from build123d import *

# Parameters (mm, degrees)
F1_DEPTH  = 74.8970308
F2_R      = 1.35255
F3_DEPTH  = 1.70942
F8_DEPTH  = 150.2936248359
F10_DEPTH = 91.0812758
F11_R     = 3.69315
F12_R     = 1.98373
F12_R_2   = 1.98374
F13_R     = 0.762


# Not quite as in the source:
# - a fillet or chamfer is up to 0.001 mm smaller than in the source, because OpenCascade refuses the exact size


with BuildPart() as f1:
    # F0 (on Top) → F1 (new body)
    with BuildSketch(Plane.XY):
        Polygon((0, -34.9127429517), (0, 0), (4.6326774961, 3.932751029), (7.9712502047, 0), (9.2744217668, 1.1062823402), (4.8295667179, 6.3422049313), (-1.70942, 0.7911587457), (-1.70942, -36.6221629517), (155.9705248359, -36.6221629517), (155.9705248359, 0.7911587457), (149.4315381179, 6.3422049313), (144.9866830691, 1.1062823402), (146.2898546311, 0), (149.6284273398, 3.932751029), (154.2611048359, 0), (154.2611048359, -34.9127429517), align=None)
    extrude(amount=F1_DEPTH)

    # F2 (on face) → F3 (cut, through all)
    with BuildSketch(Plane(origin=(0, -34.9127429517, 0), x_dir=(-1, 0, 0), z_dir=(0, 1, 0))):
        with Locations((-5.15874, 3.175)):
            Circle(F2_R)
        with Locations((-5.15874, 63.2981208)):
            Circle(F2_R)
        with Locations((-149.1023648359, 63.2981208)):
            Circle(F2_R)
        with Locations((-149.1023648359, 3.175)):
            Circle(F2_R)
    extrude(amount=-F3_DEPTH, mode=Mode.SUBTRACT)

    # F7 (on offset) → F8 (join, through all)
    with BuildSketch(Plane.YZ.offset(1.98374)):
        with BuildLine():
            Line((-36.6221629517, 74.8970308), (-34.9127429517, 74.8970308))
            ThreePointArc((-34.9127429517, 74.8970308), (-35.0846656967, 76.2029136969), (-35.5887176805, 77.4198028324))
            Line((-35.5887176805, 77.4198028324), (-81.129350806, 156.2984932146))
            Line((-81.129350806, 156.2984932146), (-82.6097519517, 155.4437832146))
            Line((-82.6097519517, 155.4437832146), (-37.0691188262, 76.5650928324))
            ThreePointArc((-37.0691188262, 76.5650928324), (-36.7358386226, 75.7604832448), (-36.6221629517, 74.8970308))
        make_face()
    extrude(amount=F8_DEPTH)

    # F9 (on face) → F10 (join)
    with BuildSketch(Plane(origin=(0, -87.96157055, 152.3539093062), x_dir=(1, 0, 0), z_dir=(0, -0.5, 0.8660254038))):
        Polygon((-1.7094199999, 6.1797478168), (1.98374, 6.1797478168), (1.98374, 7.8891678168), (0, 7.8891678168), (1e-10, 28.9964815425), (4.3557372213, 33.3522187635), (8.0035172575, 29.7044387269), (9.2122597315, 30.9131812007), (4.3557372215, 35.7697037112), (-1.7094199999, 29.7045464903), align=None)
        Polygon((152.277364836, 7.8891678168), (152.277364836, 6.1797478168), (155.9705248359, 6.1797478168), (155.9705248359, 29.7045464903), (149.9053676148, 35.7697037114), (145.0488451045, 30.9131812012), (146.2575875784, 29.7044387273), (149.9053676148, 33.3522187636), (154.2611048359, 28.9964815425), (154.2611048359, 7.8891678168), align=None)
    extrude(amount=-F10_DEPTH)

    # F11 (radius 3.69316 in the source; OpenCascade refuses exactly that, so slightly less here)
    f11_edges = [f1.edges().sort_by_distance(p)[0] for p in [
        (149.431538, 6.342205, 37.448515),
        (155.970525, 0.791159, 37.448515),
        (155.970525, -36.622163, 37.448515),
        (-1.70942, -36.622163, 37.448515),
        (-1.70942, 0.791159, 37.448515),
        (4.829567, 6.342205, 37.448515),
        (149.905368, -34.21378, 130.799412),
        (155.970525, -39.46636, 127.766833),
        (155.970525, -59.839433, 116.004434),
        (-1.70942, -59.839433, 116.004434),
        (-1.70942, -39.46636, 127.766833),
        (4.355737, -34.21378, 130.799412),
    ]]
    fillet(f11_edges, radius=F11_R)

    # F12#9 (call 1 of 12: OpenCascade refuses the feature's edges together) (radius 1.98374 in the source; OpenCascade refuses exactly that, so slightly less here)
    f12_9_edges = [f1.edges().sort_by_distance(p)[0] for p in [
        (0, -58.359032, 116.859144),
    ]]
    fillet(f12_9_edges, radius=F12_R)

    # F12#10 (call 2 of 12) (radius 1.98374 in the source; OpenCascade refuses exactly that, so slightly less here)
    f12_10_edges = [f1.edges().sort_by_distance(p)[0] for p in [
        (154.261105, -58.359032, 116.859144),
    ]]
    fillet(f12_10_edges, radius=F12_R)

    # F12#11 (call 3 of 12)
    f12_11_edges = [f1.edges().sort_by_distance(p)[0] for p in [
        (154.261105, -40.079562, 127.412801),
    ]]
    fillet(f12_11_edges, radius=F12_R_2)

    # F12#12 (call 4 of 12)
    f12_12_edges = [f1.edges().sort_by_distance(p)[0] for p in [
        (149.905368, -36.307383, 129.590669),
    ]]
    fillet(f12_12_edges, radius=F12_R_2)

    # F12 (call 5 of 12)
    f12_edges = [f1.edges().sort_by_distance(p)[0] for p in [
        (149.628427, 3.932751, 37.448515),
    ]]
    fillet(f12_edges, radius=F12_R_2)

    # F12#2 (call 6 of 12)
    f12_2_edges = [f1.edges().sort_by_distance(p)[0] for p in [
        (154.261105, 0, 37.448515),
    ]]
    fillet(f12_2_edges, radius=F12_R_2)

    # F12#3 (call 7 of 12)
    f12_3_edges = [f1.edges().sort_by_distance(p)[0] for p in [
        (154.261105, -34.912743, 37.448515),
    ]]
    fillet(f12_3_edges, radius=F12_R_2)

    # F12#4 (call 8 of 12)
    f12_4_edges = [f1.edges().sort_by_distance(p)[0] for p in [
        (0, -34.912743, 37.448515),
    ]]
    fillet(f12_4_edges, radius=F12_R_2)

    # F12#5 (call 9 of 12)
    f12_5_edges = [f1.edges().sort_by_distance(p)[0] for p in [
        (0, 0, 37.448515),
    ]]
    fillet(f12_5_edges, radius=F12_R_2)

    # F12#6 (call 10 of 12)
    f12_6_edges = [f1.edges().sort_by_distance(p)[0] for p in [
        (4.632677, 3.932751, 37.448515),
    ]]
    fillet(f12_6_edges, radius=F12_R_2)

    # F12#7 (call 11 of 12)
    f12_7_edges = [f1.edges().sort_by_distance(p)[0] for p in [
        (0, -40.079562, 127.412801),
    ]]
    fillet(f12_7_edges, radius=F12_R_2)

    # F12#8 (call 12 of 12)
    f12_8_edges = [f1.edges().sort_by_distance(p)[0] for p in [
        (4.355737, -36.307383, 129.590669),
    ]]
    fillet(f12_8_edges, radius=F12_R_2)

    # F13
    f13_edges = [f1.edges().sort_by_distance(p)[0] for p in [
        (145.638269, 0.553141, 74.897031),
        (145.638269, 0.553141, 0),
        (8.622836, 0.553141, 0),
        (8.622836, 0.553141, 74.897031),
        (8.607888, -61.713371, 167.508314),
        (8.607888, -16.172733, 88.629616),
        (145.653216, -16.172733, 88.629616),
        (145.653216, -61.713371, 167.508314),
    ]]
    fillet(f13_edges, radius=F13_R)


solid = f1.part
Can you work these out from the model? Positions are in its coordinate system, mm. A direction names the side the tool comes from. Round coordinates to 2 decimals unless told otherwise and drop trailing zeros. Order: outer loops, then holes, each group sorted by start corner. A loop starts at its lowest first (then second) coordinate and runs counter-clockwise, first axis right, second up. Notation, with made-up numbers: M 61.5,33 L 76.5,33 A24 ccw 76.5,56 Z; hole C -7.75,54 d8. An arc over 180 degrees is marked long. Use a Markdown table: item, result.
1) Imagine slicing it at C-C (x = 110). List the corners of the cut face in (y, z) for me, then the cut area to 3 significant figures.
Geometry says:
| item | result |
|---|---|
| outline | M -82.61,155.44 L -37.07,76.57 A3.34 cw -36.62,74.9 L -36.62,0 L -34.91,0 L -34.91,74.9 A5.05 ccw -35.59,77.42 L -81.13,156.3 Z |
| area | 287 mm² |
2) If we mould it in two halves opening along Z, with no side actions, what happens to faces 4 (the face through (-0.6, -58.61, 115.98)), 5 (the face through (154.261, -49, 123)), 6 (the face through (0, -49, 123)), 7 (the face through (154.261, -17, 37))? For each: +Z half, -Z half, draft (parallel to the pull), parting line (faces both ways), or undercut.
Geometry says:
| item | result |
|---|---|
| face 4 | -Z half |
| face 5 | undercut |
| face 6 | undercut |
| face 7 | draft |
3) Imagine slicing it at A-A (z = 35). List the corners of the cut face in (x, y) for me, then the cut area to 3 significant figures.
Geometry says:
| item | result |
|---|---|
| outline | M -1.71,-32.93 A3.69 ccw 1.98,-36.62 L 152.28,-36.62 A3.69 ccw 155.97,-32.93 L 155.97,-0.92 A3.69 ccw 154.67,1.9 L 152.25,3.95 A3.69 ccw 147.04,3.53 L 144.99,1.11 L 146.29,0 L 148.34,2.42 A1.98 cw 151.14,2.65 L 153.56,0.59 A1.98 cw 154.26,-0.92 L 154.26,-32.93 A1.98 cw 152.28,-34.91 L 1.98,-34.91 A1.98 cw 0,-32.93 L 0,-0.92 A1.98 cw 0.7,0.59 L 3.12,2.65 A1.98 cw 5.92,2.42 L 7.97,0 L 9.27,1.11 L 7.22,3.53 A3.69 ccw 2.01,3.95 L -0.41,1.9 A3.69 ccw -1.71,-0.92 Z |
| area | 427 mm² |
4) On a 3-axis mill with a long thin cutter (end or side, diameter ignored), from which of +Z, -Z, +X, -X, +Y, -Y can I reach the whole of each face in a straight line? I mean faces 1 (the face through (8.105, -37.78, 129.477)), 2 (the face through (152.477, -38.854, 128.857)), 3 (the face through (-1.709, -17, 37)). Say none if no direction works.
Geometry says:
| item | result |
|---|---|
| face 1 | +Z, +Y |
| face 2 | none |
| face 3 | +Z, -Z, -X, +Y, -Y |
5) Imagine slicing it at B-B (y = -9). List the corners of the cut face in (x, z) for me, then the cut area to 3 significant figures.
Geometry says:
| item | result |
|---|---|
| outline | M -1.71,0 L 0,0 L 0,74.9 L -1.71,74.9 Z; M 154.26,0 L 155.97,0 L 155.97,74.9 L 154.26,74.9 Z |
| area | 256 mm² |
6) I'm going to push flat-ended pins straight in: P1, Ø3, axis at x = 76, y = -56, coming from the +Z side; P2, Ø5, axis at x = 150.5, y = -19, coming from the +Z side; P3, Ø1.1, axis at y = -36, z = 76, coming from the +X side. Where does each tip first touch, or does it pass through?
Geometry says:
| item | result |
|---|---|
| P1 | stops at z = 115.37 |
| P2 | stops at z = 105.67 |
| P3 | stops at x = 152.28 |
7) If I drill on line 1 along X through (y, z) = (-6, 30.5); line 2 along Y through (x, z) = (91.5, 25.5); line 3 along Y through (x, z) = (98.5, 134), over which ranges is the centre line in solid material (lowest first)?
Geometry says:
| item | result |
|---|---|
| line 1 | x = -1.71 to 0, 154.26 to 155.97 |
| line 2 | y = -36.62 to -34.91 |
| line 3 | y = -70.23 to -68.26 |
